```python
from build123d import *

# Parameters (mm, degrees)
F0_R     = 1.95
F0_R_2   = 3.3
F0_R_3   = 1.75
F1_DEPTH = 8.8
F2_DEPTH = 3.5
F3_DEPTH = 3.5
F4_SIZE  = 0.3
F5_R     = 0.5


with BuildPart() as f1:
    # F0 (on Front) → F1 (new body)
    with BuildSketch(Plane.XZ):
        Polygon((28.8, -3.783914), (-11.2, -3.783914), (-11.2, -12.183914), (-4.2, -12.183914), (-4.2, -22.183914), (21.8, -22.183914), (21.8, -12.183914), (28.8, -12.183914), align=None)
        with Locations((8.7, -18.783914)):
            Circle(F0_R, mode=Mode.SUBTRACT)
        with Locations((0, -8.783914)):
            Circle(F0_R_2, mode=Mode.SUBTRACT)
        with Locations((5.8, -8.783914)):
            Circle(F0_R, mode=Mode.SUBTRACT)
        with Locations((11.6, -8.783914)):
            Circle(F0_R, mode=Mode.SUBTRACT)
        with Locations((17.6, -8.783914)):
            Circle(F0_R_2, mode=Mode.SUBTRACT)
        with Locations((0, -8.783914)):
            Circle(F0_R_2)
        with Locations((0, -8.783914)):
            Circle(F0_R_3, mode=Mode.SUBTRACT)
        with Locations((17.6, -8.783914)):
            Circle(F0_R_2)
        with Locations((17.6, -8.783914)):
            Circle(F0_R_3, mode=Mode.SUBTRACT)
        with Locations((11.6, -8.783914)):
            Circle(F0_R)
        with Locations((11.6, -8.783914)):
            Circle(F0_R_3, mode=Mode.SUBTRACT)
        with Locations((5.8, -8.783914)):
            Circle(F0_R)
        with Locations((5.8, -8.783914)):
            Circle(F0_R_3, mode=Mode.SUBTRACT)
        with Locations((8.7, -18.783914)):
            Circle(F0_R)
        with Locations((8.7, -18.783914)):
            Circle(F0_R_3, mode=Mode.SUBTRACT)
    extrude(amount=-F1_DEPTH)

    # F0 (on Front) → F2 (cut)
    with BuildSketch(Plane.XZ):
        with Locations((17.6, -8.783914)):
            Circle(F0_R_2)
        with Locations((17.6, -8.783914)):
            Circle(F0_R_3, mode=Mode.SUBTRACT)
    extrude(amount=-F2_DEPTH, mode=Mode.SUBTRACT)

    # F0 (on Front) → F3 (cut)
    with BuildSketch(Plane.XZ):
        with Locations((0, -8.783914)):
            Circle(F0_R_2)
        with Locations((0, -8.783914)):
            Circle(F0_R_3, mode=Mode.SUBTRACT)
    extrude(amount=-F3_DEPTH, mode=Mode.SUBTRACT)

    # F4
    f4_edges = [f1.edges().sort_by_distance(p)[0] for p in [
        (9.85, 8.8, -8.783914),
        (4.05, 8.8, -8.783914),
        (6.95, 8.8, -18.783914),
    ]]
    chamfer(f4_edges, length=F4_SIZE)

    # F5
    f5_edges = [f1.edges().sort_by_distance(p)[0] for p in [
        (-11.2, 4.4, -3.783914),
        (-11.2, 4.4, -12.183914),
        (-4.2, 4.4, -22.183914),
        (28.8, 4.4, -12.183914),
        (28.8, 4.4, -3.783914),
        (21.8, 4.4, -22.183914),
    ]]
    fillet(f5_edges, radius=F5_R)


solid = f1.part
```
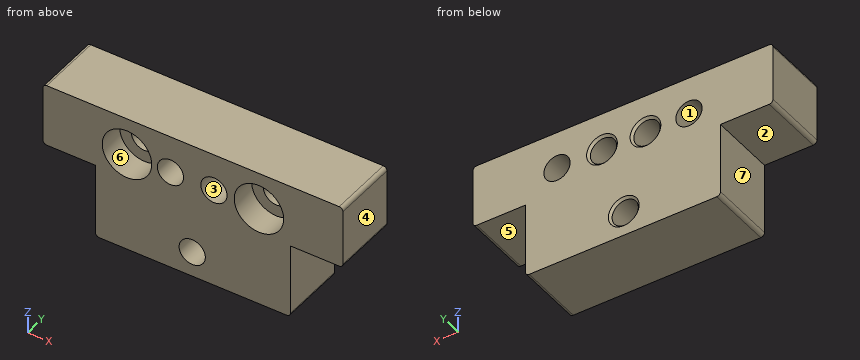
Check sheet for the modelled part. Datum: model origin and axes. Units: mm. Face numbers are marked on the shaded views. A direction names the side the tool comes from. Round coordinates to 2 decimals unless told otherwise and drop trailing zeros. Order: outer loops, then holes, each group sorted by start corner. A loop starts at its lowest first (then second) coordinate and runs counter-clockwise, first axis right, second up. Notation, with made-up numbers: (26.5, 46.5) - (64.5, 46.5) arc R9 ccw to (64.5, 55.5) - close; hole circle Ø6 at (-30, 17). An arc over 180 degrees is marked (long way). Answer as CSV lines item,"result". Start each with the question number.
1) Draft check along X on the marked faces 1, 2, 3 and 4. Enter one of: +X half, -X half, draft (parallel to the pull), parting line (faces both ways), or undercut.
2) Section check D-D (z = -13.25). Record the cut outline in (x, y).
3) Tool access check on the marked faces 5, 6 and 7. Record the directions out of +Z, -Z, +X, -X, +Y, -Y that give a thin tool (end or side, any length) a straight path to the whole face; none if there is none.
4) Section check B-B (y = 7.5). Record the cut outline in (x, z).
5) Depth check by flat-ended pin: pin 1 (1.9 mm diameter, centred on x = -6, y = 3, fed in from -Z); pin 2 (2.5 mm diameter, centred on y = 5.5, z = -14.5, fed in from +X); pin 3 (4 mm diameter, centred on x = 0, z = -8.78, fed in from -Y); pin 4 (3 mm diameter, centred on x = 17.6, z = -8.78, fed in from -Y). Enter the tip coordinate at first touch or a pass-through.
6) Scan lines: probe 1 along Z at (x, y) = (0, 1.55); probe 2 along X at (y, z) = (1.5, -6.5); probe 3 along X at (y, z) = (3, -7). Record each from-to range of solid material in increasing order.
7) Section check C-C (x = 11.6). Record the cut outline in (y, z), then the cut area to 3 significant figures.
8) Section check A-A (x = 17.6). Record the cut outline in (y, z), then the cut area to 3 significant figures.
Determined:
1,face 1,"undercut"
1,face 2,"draft"
1,face 3,"undercut"
1,face 4,"+X half"
2,outline,"(-4.2, 0) - (21.8, 0) - (21.8, 8.8) - (-4.2, 8.8) - close"
3,face 5,"-Z, +X, +Y, -Y"
3,face 6,"-Y"
3,face 7,"-Z, -X, +Y, -Y"
4,outline,"(-11.2, -11.68) arc R0.5 ccw to (-10.7, -12.18) - (-4.2, -12.18) - (-4.2, -21.68) arc R0.5 ccw to (-3.7, -22.18) - (21.3, -22.18) arc R0.5 ccw to (21.8, -21.68) - (21.8, -12.18) - (28.3, -12.18) arc R0.5 ccw to (28.8, -11.68) - (28.8, -4.28) arc R0.5 ccw to (28.3, -3.78) - (-10.7, -3.78) arc R0.5 ccw to (-11.2, -4.28) - close; hole circle Ø3.5 at (0, -8.78); hole circle Ø3.5 at (5.8, -8.78); hole circle Ø3.5 at (8.7, -18.78); hole circle Ø3.5 at (11.6, -8.78); hole circle Ø3.5 at (17.6, -8.78)"
5,pin 1,"z = -12.18"
5,pin 2,"x = 21.8"
5,pin 3,"y = 3.5"
5,pin 4,"through"
6,probe 1,"-22.18 to -12.08, -5.48 to -3.78"
6,probe 2,"-11.2 to -2.38, 2.38 to 15.22, 19.98 to 28.8"
6,probe 3,"-11.2 to -2.78, 2.78 to 14.82, 20.38 to 28.8"
7,outline,"(0, -22.18) - (8.8, -22.18) - (8.8, -10.83) - (8.5, -10.53) - (0, -10.53) - close; (0, -7.03) - (8.5, -7.03) - (8.8, -6.73) - (8.8, -3.78) - (0, -3.78) - close"
7,area,"131 mm^2"
8,outline,"(0, -22.18) - (8.8, -22.18) - (8.8, -10.53) - (3.5, -10.53) - (3.5, -12.08) - (0, -12.08) - close; (0, -5.48) - (3.5, -5.48) - (3.5, -7.03) - (8.8, -7.03) - (8.8, -3.78) - (0, -3.78) - close"
8,area,"120 mm^2"
